Work out the finished part from the listing and answer in its coordinate system (mm). A direction names the side the tool comes from. Round coordinates to 2 decimals unless told otherwise and drop trailing zeros. Write each loop counter-clockwise with the first axis right and the second up, starting at its lowest first coordinate (ties: lowest second). Pieces come first, ordered by that corner, then holes.
1. Flat-ended cylindrical pins translate along their axes: pin 1 Ø10 at (x, z) = (109, 53.5) entering from +Y; pin 2 Ø19 at (x, z) = (-780.5, 64) entering from +Y; pin 3 Ø19 at (y, z) = (64, 73) entering from +X. Find the tip coordinate at first contact, or state that the pin passes through.
2. Straight lines are drawn through the part: probe 1 along Z at (x, y) = (-524, 89.5); probe 2 along Y at (x, z) = (-717.5, 34.5); probe 3 along X at (y, z) = (62.5, 106). For each, find the intervals that lie inside material, in ascending order.
3. Determine the mould class of faces 1 (the face through (800.1, 50, 6)), 2 (the face through (4, 101.6, -399)), 3 (the face through (781.32, 76.56, -158.66)) for opening direction X: pulls with the +X half, pulls with the -X half, needs draft (parallel to the pull), parting line crosses it, or undercut.
4. Find section B-B (x = -134). Write down the section's boundary in (y, z).
5. Find section A-A (z = 245). Write down the section's boundary in (x, y).
6. A tool of negligible diameter and unlimited length cuts with its end or side. For faces 4 (the face through (-743.892, 95.161, 361.905)), 5 (the face through (-11, 50, 412.75)), from which of +Z, -Z, +X, -X, +Y, -Y can it reach the whole face along a straight path? Write none if from no direction.
```python
from build123d import *

# Parameters (mm, degrees)
SKETCH5_W           = 1600.2
SKETCH5_H           = 825.5
BOSS_EXTRUDE1_DEPTH = 101.6
SKETCH6_W           = 1524
SKETCH6_H           = 762
CUT_EXTRUDE1_DEPTH  = 12.7
CUT_EXTRUDE2_DEPTH  = 50.8
CUT_EXTRUDE3_DEPTH  = 50.8
BOSS_EXTRUDE4_DEPTH = 12.7


with BuildPart() as part:
    # Sketch5 → Boss-Extrude1 (new body)
    with BuildSketch(Plane(origin=(0, 0, 0), x_dir=(1, 0, 0), z_dir=(0, 1, 0))):
        Rectangle(SKETCH5_W, SKETCH5_H)
    extrude(amount=BOSS_EXTRUDE1_DEPTH)

    # Sketch6 → Cut-Extrude1 (cut)
    with BuildSketch(Plane(origin=(0, 101.6, 0), x_dir=(1, 0, 0), z_dir=(0, 1, 0))):
        Rectangle(SKETCH6_W, SKETCH6_H)
    extrude(amount=-CUT_EXTRUDE1_DEPTH, mode=Mode.SUBTRACT)

    # Sketch10 → Cut-Extrude2 (cut)
    with BuildSketch(Plane(origin=(0, 101.6, 0), x_dir=(1, 0, 0), z_dir=(0, 1, 0))):
        Polygon((800.1, -152.4), (800.1, 0), (800.1, 152.4), (762, 165.1), (762, 0), (762, -165.1), align=None)
    extrude(amount=-CUT_EXTRUDE2_DEPTH, mode=Mode.SUBTRACT)

    # Sketch12 → Cut-Extrude3 (cut)
    with BuildSketch(Plane(origin=(0, 101.6, 0), x_dir=(1, 0, 0), z_dir=(0, 1, 0))):
        Polygon((-800.1, 0), (-800.1, 152.4), (-762, 165.1), (-762, 0), (-762, -165.1), (-800.1, -152.4), align=None)
    extrude(amount=-CUT_EXTRUDE3_DEPTH, mode=Mode.SUBTRACT)

    # Sketch16 → Boss-Extrude4 (add)
    with BuildSketch(Plane(origin=(0, 88.9, 0), x_dir=(1, 0, 0), z_dir=(0, 1, 0))):
        with BuildLine():
            Line((762, 381), (762, 317.5))
            ThreePointArc((762, 317.5), (743.401280605, 362.401280605), (698.5, 381))
            Line((698.5, 381), (762, 381))
        make_face()
        with BuildLine():
            Line((-762, 317.5), (-762, 381))
            Line((-762, 381), (-698.5, 381))
            ThreePointArc((-698.5, 381), (-743.401280605, 362.401280605), (-762, 317.5))
        make_face()
        with BuildLine():
            Line((-698.5, -381), (-762, -381))
            Line((-762, -381), (-762, -317.5))
            ThreePointArc((-762, -317.5), (-743.401280605, -362.401280605), (-698.5, -381))
        make_face()
        with BuildLine():
            Line((698.5, -381), (762, -381))
            Line((762, -381), (762, -317.5))
            ThreePointArc((762, -317.5), (743.401280605, -362.401280605), (698.5, -381))
        make_face()
    extrude(amount=BOSS_EXTRUDE4_DEPTH)


solid = part.part
```
Worked answers:
1. pin 1: stops at y = 88.9
1. pin 2: stops at y = 50.8
1. pin 3: stops at x = 762
2. probe 1: z = -412.75 to -381, 381 to 412.75
2. probe 2: y = 0 to 88.9
2. probe 3: x = -762 to 762
3. face 1: pulls with the +X half
3. face 2: needs draft
3. face 3: undercut
4. outline: (0, -412.75) - (101.6, -412.75) - (101.6, -381) - (88.9, -381) - (88.9, 381) - (101.6, 381) - (101.6, 412.75) - (0, 412.75) - close
5. outline: (-800.1, 0) - (800.1, 0) - (800.1, 101.6) - (762, 101.6) - (762, 88.9) - (-762, 88.9) - (-762, 101.6) - (-800.1, 101.6) - close
6. face 4: +Y
6. face 5: +Z, +X, -X, +Y, -Y
